Design review of the part built by this model. Coordinates are the model's own, in mm. A direction names the side the tool comes from. Give positions to 0.01 mm unless a question says otherwise; leave off trailing zeros. Order: outer loops, then holes, each group sorted by start corner. A loop starts at its lowest first (then second) coordinate and runs counter-clockwise, first axis right, second up.
```python
from build123d import *

# Parameters (mm, degrees)
BOSS_EXTRUDE1_DEPTH   = 30.9
F_5_0MM_DOWEL_HOLE1_D = 5


with BuildPart() as part:
    # Sketch1 → Boss-Extrude1 (new body)
    with BuildSketch(Plane.XY):
        Polygon((3, 0), (133, 0), (133, -90), (136, -90), (156, -90), (156, -87), (136, -87), (136, 0), (136, 3), (0, 3), (0, 0), (0, -87), (-20, -87), (-20, -90), (0, -90), (3, -90), align=None)
    extrude(amount=BOSS_EXTRUDE1_DEPTH)

    # Ø5.0mm Dowel Hole1 (through all)
    with Locations(Plane(origin=(0, -87, 0), x_dir=(1, 0, 0), z_dir=(0, 1, 0))):
        with Locations((-10, -15), (146, -15)):
            Hole(F_5_0MM_DOWEL_HOLE1_D / 2)


solid = part.part
```
1. Draft analysis for pull direction X (two halves, no side actions). For faces 1 (the face through (146, -87, 12)), 2 (the face through (67, 0, 15)), 3 (the face through (0, -41, 15)), state which applies: pulls with the +X half, pulls with the -X half, needs draft (parallel to the pull), parting line crosses it, or undercut.
Recorded:
face 1: needs draft
face 2: undercut
face 3: pulls with the -X half
2. Take a section at C-C (y = -17). State the section outline as (x, z) points.
Recorded:
outline: (0, 0) - (3, 0) - (3, 30.9) - (0, 30.9) - close; (133, 0) - (136, 0) - (136, 30.9) - (133, 30.9) - close
3. Take a section at B-B (x = -10). State the section outline as (y, z) points, then the cut area to 3 significant figures.
Recorded:
outline: (-90, 0) - (-87, 0) - (-87, 12.5) - (-90, 12.5) - close; (-90, 17.5) - (-87, 17.5) - (-87, 30.9) - (-90, 30.9) - close
area: 77.7 mm2
4. Take a section at A-A (z = 15). State the section outline as (x, y) points, then the cut area to 3 significant figures.
Recorded:
outline: (-20, -90) - (-12.5, -90) - (-12.5, -87) - (-20, -87) - close; (-7.5, -90) - (3, -90) - (3, 0) - (133, 0) - (133, -90) - (143.5, -90) - (143.5, -87) - (136, -87) - (136, 3) - (0, 3) - (0, -87) - (-7.5, -87) - close; (148.5, -90) - (156, -90) - (156, -87) - (148.5, -87) - close
area: 1,040 mm2
5. Machinability: for faces 4 (the face through (35, 1, 0)), 5 (the face through (133, -44, 15)), 6 (the face through (35, 1, 30.9)), 7 (the face through (136, -43, 15)), 8 (the face through (-10, -87, 12)), which of the approach directions +Z, -Z, +X, -X, +Y, -Y give a long, thin tool a straight path to every point of the face, cutting with its end or side? Answer none if there is none.
Recorded:
face 4: -Z, +X, -X, +Y, -Y
face 5: +Z, -Z, -Y
face 6: +Z, +X, -X, +Y, -Y
face 7: +Z, -Z, +X, +Y
face 8: +Z, -Z, -X, +Y
6. Take a section at D-D (z = 28). State the section outline as (x, y) points.
Recorded:
outline: (-20, -90) - (3, -90) - (3, 0) - (133, 0) - (133, -90) - (156, -90) - (156, -87) - (136, -87) - (136, 3) - (0, 3) - (0, -87) - (-20, -87) - close
7. For pin 1 (2 mm diameter, centred on x = 98.5, z = 7.5, fed in from -Y); pin 2 (15.5 mm diameter, centred on y = -62.5, z = 14, fed in from -X); pin 3 (16 mm diameter, centred on x = 142, z = 21, fed in from +Y); pin 4 (6.5 mm diameter, centred on x = 146, z = 15, fed in from +Y), all flat-tipped, find the tip position at first contact; note any pin that passes through.
Recorded:
pin 1: stops at y = 0
pin 2: stops at x = 0
pin 3: stops at y = 3
pin 4: stops at y = -87
8. For line 1 along X through (y, z) = (-88, 15); line 2 along X through (y, z) = (-46, 20); line 3 along Z through (x, y) = (-10, -89.3), list the stretches that pass through material, from the lowest coordinate up.
Recorded:
line 1: x = -20 to -12.5, -7.5 to 3, 133 to 143.5, 148.5 to 156
line 2: x = 0 to 3, 133 to 136
line 3: z = 0 to 12.5, 17.5 to 30.9
